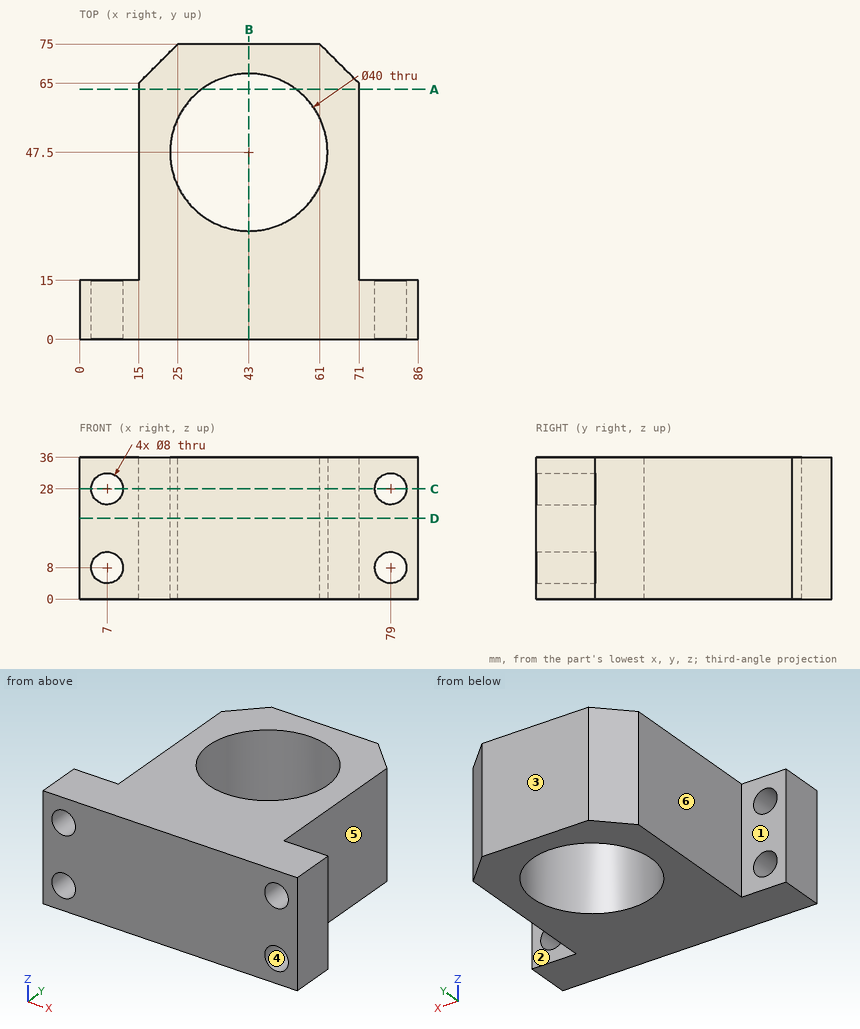
Here's the drawing with two shaded views (mm, measured from the low corner). I have some questions. A direction names the side the tool comes from. Give positions to 0.01 mm unless a question says otherwise; leave off trailing zeros. Loops run counter-clockwise (first coordinate to the right, second up) from the corner with the lowest first, then second, coordinate; pieces in that order, holes last. Notation, with made-up numbers: M 57.5,-9.5 L 71.5,-9.5 A20 ccw 71.5,2.5 Z; hole C 52,16.5 d10. An arc over 180 degrees is marked long. One line per item, written item: value. Start each with the question number.
1) If we section it at A-A, the plane y = 63.5: Write out the boundary of the cut face in (x, z), and give its area (3 significant figures).
2) Thinking about a two-plate mould opening in X: for the marked faces 4, 5 and 6, which applies, +X half, -X half, draft (parallel to the pull), parting line (faces both ways), or undercut?
3) If we section it at D-D, the plane z = 20.5: Write out the boundary of the cut face in (x, y), and give its area (3 significant figures).
4) If I drill on line 1 (X direction, y = 3, z = 8); line 2 (Z direction, x = 79, y = 11); line 3 (Y direction, x = 43, z = 16), over which ranges is the centre line in solid material (lowest first)? Write a range as [from, to].
5) If we section it at C-C, the plane z = 28: Write out the boundary of the cut face in (x, y).
6) If we section it at B-B, the plane x = 43: Write out the boundary of the cut face in (y, z).
7) On a 3-axis mill with a long thin cutter (end or side, diameter ignored), from which of +Z, -Z, +X, -X, +Y, -Y can I reach the whole of each face in a straight line? I mean the marked faces 1, 2 and 3. Say none if no direction works.
8) I'm going to push flat-ended pins straight in: pin 1 (5 mm diameter, centred on y = 15.5, z = 29, fed in from -X); pin 2 (18 mm diameter, centred on y = 43, z = 23, fed in from +X); pin 3 (10 mm diameter, centred on x = 70.5, z = 5.5, fed in from +Y); pin 4 (3 mm diameter, centred on x = 35, y = 32.5, fed in from +Z). Where does each tip first touch, or does it pass through?
Completed:
1. outline: M 15,0 L 31,0 L 31,36 L 15,36 Z; M 55,0 L 71,0 L 71,36 L 55,36 Z
1. area: 1,150 mm^2
2. face 4: undercut
2. face 5: +X half
2. face 6: -X half
3. outline: M 0,0 L 86,0 L 86,15 L 71,15 L 71,65 L 61,75 L 25,75 L 15,65 L 15,15 L 0,15 Z; hole C 43,47.5 d40
3. area: 3,290 mm^2
4. line 1: x = [0, 3], [11, 75], [83, 86]
4. line 2: z = [0, 4], [12, 24], [32, 36]
4. line 3: y = [0, 27.5], [67.5, 75]
5. outline: M 0,0 L 3,0 L 3,15 L 0,15 Z; M 11,0 L 75,0 L 75,15 L 71,15 L 71,65 L 61,75 L 25,75 L 15,65 L 15,15 L 11,15 Z; M 83,0 L 86,0 L 86,15 L 83,15 Z; hole C 43,47.5 d40
6. outline: M 0,0 L 27.5,0 L 27.5,36 L 0,36 Z; M 67.5,0 L 75,0 L 75,36 L 67.5,36 Z
7. face 1: +Z, -Z, -X, +Y
7. face 2: +Z, -Z, +X, +Y
7. face 3: +Z, -Z, +X, -X, +Y
8. pin 1: stops at x = 0
8. pin 2: stops at x = 71
8. pin 3: stops at y = 70.5
8. pin 4: passes through
